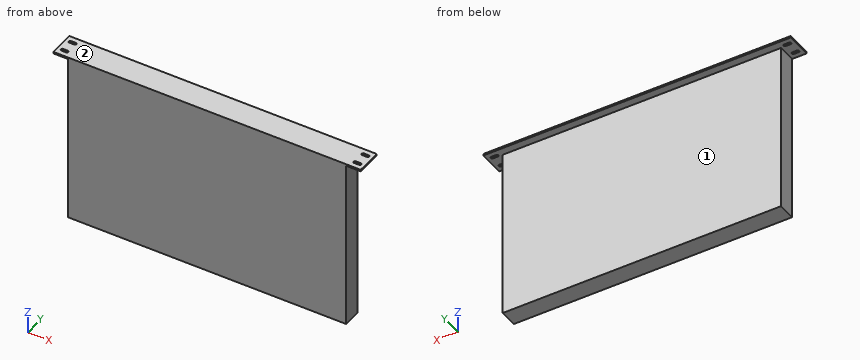
Autodesk Inventor part; units mm, degrees
ref_plane "YZ Plane" through (0, 0, 0) normal (1, 0, 0) x (0, 1, 0)
ref_plane "XZ Plane" through (0, 0, 0) normal (0, 1, 0) x (-1, 0, 0)
ref_plane "XY Plane" through (0, 0, 0) normal (0, 0, 1) x (1, 0, 0)
sketch "Sketch1" plane through (0, 0, 0) normal (0, 0, 1) x (1, 0, 0)
  line L0 (-241.3, -20.193) -> (241.3, -20.193)
  line L1 (241.3, -20.193) -> (241.3, 20.193)
  line L2 (241.3, 20.193) -> (-241.3, 20.193)
  line L3 (-241.3, 20.193) -> (-241.3, -20.193)
  line L4 (-241.3, -20.193) -> (241.3, 20.193) construction
  line L5 (241.3, -20.193) -> (-241.3, 20.193) construction
  point P0 (0, 0)
  dimension "d0" = 482.6
  dimension "d1" = 40.386
extrude "Extrusion1" add sketch "Sketch1" against normal blind 2.6416
sketch "Sketch2" plane through (0, 0, -2.6416) normal (0, 0, -1) x (-1, 0, 0)
  line L0 (-241.3, -20.193) -> (241.3, -20.193)
  line L1 (-218.44, -20.193) -> (218.44, -20.193)
  line L2 (218.44, -20.193) -> (218.44, 7.913)
  line L3 (218.44, 7.913) -> (-218.44, 7.913)
  line L4 (-218.44, 7.913) -> (-218.44, -20.193)
  line L5 (0, -20.193) -> (0, 20.193) construction
  line L6 (241.3, 20.193) -> (-241.3, 20.193)
  point P0 (0, 0)
  dimension "d4" = 436.88
extrude "Extrusion2" add sketch "Sketch2" along normal blind 267.1064
sketch "Sketch3" plane through (0, 0, -2.6416) normal (0, 0, -1) x (-1, 0, 0)
  line L0 (-241.3, -20.193) -> (-218.44, -20.193)
  line L1 (-229.87, -20.193) -> (-229.87, 20.193) construction
  line L2 (229.87, -20.193) -> (229.87, 20.193) construction
  line L3 (241.3, -20.193) -> (241.3, 20.193) construction
  line L4 (241.3, 20.193) -> (-241.3, 20.193) construction
  line L5 (218.44, -20.193) -> (241.3, -20.193) construction
  line L6 (-233.6311, 10.0965) -> (-226.1089, 10.0965) construction
  line L7 (-233.6311, 7.939) -> (-226.1089, 7.939)
  line L8 (-226.1089, 12.254) -> (-233.6311, 12.254)
  arc A0 (-233.6311, 12.254) -> (-233.6311, 7.939) centre (-233.6311, 10.0965) ccw
  arc A1 (-226.1089, 7.939) -> (-226.1089, 12.254) centre (-226.1089, 10.0965) ccw
  line L9 (-241.3, 0) -> (241.3, 0) construction
  line L10 (-241.3, 20.193) -> (-241.3, -20.193)
  line L11 (-233.6311, -10.0965) -> (-226.1089, -10.0965) construction
  line L12 (-233.6311, -7.939) -> (-226.1089, -7.939)
  line L13 (-226.1089, -12.254) -> (-233.6311, -12.254)
  arc A2 (-233.6311, -7.939) -> (-233.6311, -12.254) centre (-233.6311, -10.0965) ccw
  arc A3 (-226.1089, -12.254) -> (-226.1089, -7.939) centre (-226.1089, -10.0965) ccw
  line L14 (0, 20.193) -> (0, -20.193) construction
  line L15 (-218.44, -20.193) -> (218.44, -20.193)
  line L16 (233.6311, 10.0965) -> (226.1089, 10.0965) construction
  line L17 (233.6311, 7.939) -> (226.1089, 7.939)
  line L18 (226.1089, 12.254) -> (233.6311, 12.254)
  arc A4 (233.6311, 7.939) -> (233.6311, 12.254) centre (233.6311, 10.0965) ccw
  arc A5 (226.1089, 12.254) -> (226.1089, 7.939) centre (226.1089, 10.0965) ccw
  arc A6 (226.1089, -7.939) -> (226.1089, -12.254) centre (226.1089, -10.0965) ccw
  line L19 (233.6311, -10.0965) -> (226.1089, -10.0965) construction
  line L20 (233.6311, -7.939) -> (226.1089, -7.939)
  line L21 (226.1089, -12.254) -> (233.6311, -12.254)
  arc A7 (233.6311, -12.254) -> (233.6311, -7.939) centre (233.6311, -10.0965) ccw
  point P0 (0, 0)
  point P1 (-229.87, 10.0965)
  point P2 (-229.87, -10.0965)
  point P3 (229.87, 10.0965)
  point P4 (229.87, -10.0965)
  dimension "d7" = 11.43
  dimension "d8" = 10.0965
extrude "Extrusion3" cut sketch "Sketch3" against normal up to surface (2.6416 mm away)
properties part number "PatchPanel_rep"
Can you work these out from the model? Positions are in its coordinate system, mm. Face numbers are marked on the shaded views. A direction names the side the tool comes from. Give positions to 0.01 mm unless a question says otherwise; leave off trailing zeros. Loops run counter-clockwise (first coordinate to the right, second up) from the corner with the lowest first, then second, coordinate; pieces in that order, holes last. Notation, with made-up numbers: M -24,-4 L 3,-4 A14 cw 3,8 Z; hole C -8.75,79.25 d1. An arc over 180 degrees is marked long. Answer in a Markdown table with one row per item.
1. If I drill on line 1 along Y through (x, z) = (46, -53); line 2 along Z through (x, y) = (173, 14); line 3 along X through (y, z) = (-9, -67), over which ranges is the centre line in solid material (lowest first)?
Taken from the geometry:
| item | result |
|---|---|
| line 1 | y = -20.19 to 7.91 |
| line 2 | z = -2.64 to 0 |
| line 3 | x = -218.44 to 218.44 |
2. Suppose I cut it at B-B on z = -137.5. Write out the boundary of the cut face in (x, y).
Taken from the geometry:
| item | result |
|---|---|
| outline | M -218.44,-20.19 L 218.44,-20.19 L 218.44,7.91 L -218.44,7.91 Z |
3. For pin 1 Ø8.5 at (y, z) = (-12.5, -157.5) entering from +X; pin 2 Ø8.5 at (y, z) = (-11.5, -111) entering from -X; pin 3 Ø1 at (y, z) = (9, -80) entering from -X; pin 4 Ø12 at (x, z) = (-128, -41.5) entering from +Y, each with a flat end and sliding along its axis, tell me the tip position at first contact or that it passes through.
Taken from the geometry:
| item | result |
|---|---|
| pin 1 | stops at x = 218.44 |
| pin 2 | stops at x = -218.44 |
| pin 3 | passes through |
| pin 4 | stops at y = 7.91 |
4. Which directions (+Z, -Z, +X, -X, +Y, -Y) give clear straight access to the entire face, cutting with the end or side of a thin tool? Please do the marked faces 1 and 2.
Taken from the geometry:
| item | result |
|---|---|
| face 1 | -Z, +X, -X, +Y |
| face 2 | +Z, +X, -X, +Y, -Y |
5. Suppose I cut it at A-A on x = 29.5. Write out the boundary of the cut face in (y, z).
Taken from the geometry:
| item | result |
|---|---|
| outline | M -20.19,-269.75 L 7.91,-269.75 L 7.91,-2.64 L 20.19,-2.64 L 20.19,0 L -20.19,0 Z |
